from build123d import *

# Parameters (mm, degrees)
F0_W     = 82.55
F0_H     = 57.15
F0_W_2   = 76.2
F0_H_2   = 50.8
F1_DEPTH = 152.4
F2_W     = 6.35
F2_H     = 57.15
F3_DEPTH = 50.8
F4_W     = 50.8
F4_H     = 6.35
F5_DEPTH = 50.8
F7_DEPTH = 118.618
F8_W     = 50.8
F8_H     = 158.75
F9_DEPTH = 6.35


with BuildPart() as f1:
    # F0 (on Front) → F1 (new body)
    with BuildSketch(Plane.XZ):
        with Locations((3.728271, -19.37303)):
            Rectangle(F0_W, F0_H)
        with Locations((3.728271, -19.37303)):
            Rectangle(F0_W_2, F0_H_2, mode=Mode.SUBTRACT)
    extrude(amount=F1_DEPTH)

    # F2 (on face) → F3 (join)
    with BuildSketch(Plane.YZ.offset(45.003271)):
        with Locations((-3.175, -19.37303)):
            Rectangle(F2_W, F2_H)
    extrude(amount=F3_DEPTH)

    # F4 (on face) → F5 (join)
    with BuildSketch(Plane.XZ.offset(6.35)):
        with Locations((70.403271, -44.77303)):
            Rectangle(F4_W, F4_H)
        with Locations((70.403271, 6.02697)):
            Rectangle(F4_W, F4_H)
    extrude(amount=F5_DEPTH)

    # F6 (on face) → F7 (cut)
    with BuildSketch(Plane.XY.offset(9.20197)):
        Polygon((95.803271, -6.35), (45.003271, -57.15), (95.803271, -57.15), align=None)
    extrude(amount=-F7_DEPTH, mode=Mode.SUBTRACT)

    # F8 (on face) → F9 (join)
    with BuildSketch(Plane.YZ.offset(45.003271)):
        with Locations((-127, -19.37303)):
            Rectangle(F8_W, F8_H)
    extrude(amount=F9_DEPTH)


solid = f1.part
CAD build for the part. Positions are in the model's coordinates, mm. A direction names the side the tool comes from. Round coordinates to 2 decimals unless told otherwise and drop trailing zeros. Write each loop counter-clockwise with the first axis right and the second up, starting at its lowest first coordinate (ties: lowest second). Pieces come first, ordered by that corner, then holes. Notation, with made-up numbers: M 78,-36 L 87,-36 A19 ccw 87,-4 Z; hole C -3.5,85 d10. An arc over 180 degrees is marked long. Use a Markdown table: item, result. Add a question column.
1. Slice it at B-B on y = -71.5. Give the cut face in (x, z), then the cut area to 3 significant figures.
2. Slice it at A-A on z = -29. Give the cut face in (x, y).
3. Slice it at C-C on x = 1. Give the cut face in (y, z), then the cut area to 3 significant figures.
4. 3-axis set-ups, long thin cutter, end or side, ignore diameter. For faces 5 (the face through (45.003, -127, -73)), 6 (the face through (64, -26, -41.598)), 7 (the face through (-34.372, -75, -20)), 8 (the face through (-37.547, -75, -20)): which of +Z, -Z, +X, -X, +Y, -Y reach the whole face in a straight line?
5. Pull direction Y, two halves, no side cores. Call faces 1 (the face through (58, 0, -20)), 2 (the face through (48, -101.6, -20)), 3 (the face through (45.003, -53, -20)), 4 (the face through (45.003, -127, 35)): released by +Y, released by -Y, zero draft, split by the parting line, or undercut.
6. Drill centre lines: probe 1 along X at (y, z) = (-82, 5); probe 2 along Z at (x, y) = (29, -103); probe 3 along X at (y, z) = (-109.5, -30). Where is each one in solid material? Low to high.
7. Slice it at D-D on y = -123. Give the cut face in (x, z), then the cut area to 3 significant figures.
8. Flat gauge pins, fed straight in: P1, Ø3, axis at x = 48.5, z = 15, coming from the +Y side; P2, Ø12, axis at y = -33, z = -50.5, coming from the +X side; P3, Ø2, axis at x = 41, y = -32, coming from the -Z side. Where does each tip first touch, or does it go through?
Reply:
| question | item | result |
|---|---|---|
| 1 | outline | M -37.55,-47.95 L 45,-47.95 L 45,9.2 L -37.55,9.2 Z; hole M -34.37,-44.77 L 41.83,-44.77 L 41.83,6.03 L -34.37,6.03 Z |
| 1 | area | 847 mm^2 |
| 2 | outline | M -37.55,-152.4 L -34.37,-152.4 L -34.37,0 L -37.55,0 Z; M 41.83,-152.4 L 51.35,-152.4 L 51.35,-101.6 L 45,-101.6 L 45,-6.35 L 95.8,-6.35 L 95.8,0 L 41.83,0 Z |
| 3 | outline | M -152.4,-47.95 L 0,-47.95 L 0,-44.77 L -152.4,-44.77 Z; M -152.4,6.03 L 0,6.03 L 0,9.2 L -152.4,9.2 Z |
| 3 | area | 968 mm^2 |
| 4 | face 5 | -Z, -X, +Y, -Y |
| 4 | face 6 | +X |
| 4 | face 7 | +Y, -Y |
| 4 | face 8 | +Z, -Z, -X, +Y, -Y |
| 5 | face 1 | released by +Y |
| 5 | face 2 | undercut |
| 5 | face 3 | undercut |
| 5 | face 4 | zero draft |
| 6 | probe 1 | x = -37.55 to -34.37, 41.83 to 45 |
| 6 | probe 2 | z = -47.95 to -44.77, 6.03 to 9.2 |
| 6 | probe 3 | x = -37.55 to -34.37, 41.83 to 51.35 |
| 7 | outline | M -37.55,-47.95 L 45,-47.95 L 45,-98.75 L 51.35,-98.75 L 51.35,60 L 45,60 L 45,9.2 L -37.55,9.2 Z; hole M -34.37,-44.77 L 41.83,-44.77 L 41.83,6.03 L -34.37,6.03 Z |
| 7 | area | 1,850 mm^2 |
| 8 | P1 | stops at y = -101.6 |
| 8 | P2 | stops at x = 74.58 |
| 8 | P3 | stops at z = -47.95 |
